Geometry check sheet. Reference: the model listing, model coordinates, mm. A direction names the side the tool comes from. Round coordinates to 2 decimals unless told otherwise and drop trailing zeros. Loops run counter-clockwise (first coordinate to the right, second up) from the corner with the lowest first, then second, coordinate; pieces in that order, holes last. Notation, with made-up numbers: M 4.25,33 L 13.25,33 A24 cw 13.25,48 Z; hole C 40,80 d7. An arc over 180 degrees is marked long. Answer in a Markdown table with one row per item. Add a question column.
```python
from build123d import *

# Parameters (mm, degrees)
F1_DEPTH = 6
F2_R     = 3
F3_DEPTH = 4.5
F5_D     = 3.5


# Not quite as in the source:
# - ends of sketch curves that miss each other by under 0.0002 mm in the source are joined


with BuildPart() as f1:
    # F0 (on Front) → F1 (new body)
    with BuildSketch(Plane.XZ):
        with BuildLine():
            Line((14.498358, 10), (14.498358, 14))
            Line((14.498358, 14), (14.498358, 14.25))
            Line((14.498358, 14.25), (15.498358, 14.25))
            Line((15.498358, 14.25), (16.539344, 12.069217))
            ThreePointArc((16.539344, 12.069217), (16.9083128035, 11.6541918591), (17.4418, 11.5))
            Line((17.4418, 11.5), (17.998358, 11.5))
            ThreePointArc((17.998358, 11.5), (18.3519113906, 11.6464466094), (18.498358, 12))
            Line((18.498358, 12), (18.498358, 24.5))
            ThreePointArc((18.498358, 24.5), (17.9125715624, 25.9142135624), (16.498358, 26.5))
            Line((16.498358, 26.5), (14.498358, 26.5))
            ThreePointArc((14.498358, 26.5), (13.0841444376, 25.9142135624), (12.498358, 24.5))
            Line((12.498358, 24.5), (12.498358, 22.5))
            Line((12.498358, 22.5), (12.498358, -16.25))
            ThreePointArc((12.498358, -16.25), (11.9125715624, -17.6642135624), (10.498358, -18.25))
            Line((10.498358, -18.25), (8.106805, -18.25))
            ThreePointArc((8.106805, -18.25), (4.9031601399, -18.5082508473), (1.7822496797, -19.276334039))
            Line((1.7822496797, -19.276334039), (-3.290569563, -20.9672737865))
            ThreePointArc((-3.290569563, -20.9672737865), (-4.8717084961, -24.1295514929), (-1.7094308537, -25.710690554))
            Line((-1.7094308537, -25.710690554), (2.709257, -24.237795))
            ThreePointArc((2.709257, -24.237795), (5.8301671399, -23.4697108473), (9.033812, -23.21146))
            Line((9.033812, -23.21146), (19.837293, -23.21146))
            ThreePointArc((19.837293, -23.21146), (20.3091070562, -22.8769637655), (20.1496410116, -22.3210259855))
            Line((20.1496410116, -22.3210259855), (16.154532, -19.124939))
            ThreePointArc((16.154532, -19.124939), (15.8900609581, -19.0948301233), (15.748358, -19.320156))
            Line((15.748358, -19.320156), (15.748358, -21.25))
            Line((15.748358, -21.25), (8.593639, -21.25))
            ThreePointArc((8.593639, -21.25), (5.3899932959, -21.5082508219), (2.2690829797, -22.276333939))
            Line((2.2690829797, -22.276333939), (-1.630813, -23.576299))
            ThreePointArc((-1.630813, -23.576299), (-2.263268599, -23.260072033), (-1.947040883, -22.627616351))
            Line((-1.947040883, -22.627616351), (2.106805, -21.276334))
            ThreePointArc((2.106805, -21.276334), (5.2277158277, -20.5082508979), (8.431361, -20.25))
            Line((8.431361, -20.25), (13.498358, -20.25))
            ThreePointArc((13.498358, -20.25), (14.2054647812, -19.9571067812), (14.498358, -19.25))
            Line((14.498358, -19.25), (14.498358, 10))
        make_face()
    extrude(amount=F1_DEPTH)

    # F2 (on face) → F3 (join)
    with BuildSketch(Plane.YZ.offset(14.498358)):
        with Locations((-3, -1.25)):
            Circle(F2_R)
    extrude(amount=F3_DEPTH)

    # F5 (through all)
    with Locations(Plane.YZ.offset(18.998358)):
        with Locations((-3, -1.25)):
            Hole(F5_D / 2)


solid = f1.part
```
1) Cross-section at B-B, the plane z = -6. Record the boundary of the cut face in (x, y).
2) Go/stop test with flat-tipped pins: pin 1 (1.8 mm diameter, centred on y = -3.5, z = 4, fed in from -X); pin 2 (3 mm diameter, centred on y = -2, z = -9, fed in from +X); pin 3 (1.5 mm diameter, centred on x = 12, y = -4, fed in from -Z); pin 4 (12 mm diameter, centred on x = 0.5, z = 0, fed in from +Y). Record where each tip stops, or that it passes through.
3) Cross-section at C-C, the plane x = 3.5. Record the boundary of the cut face in (y, z), plus the area to 3 significant figures.
4) Set-up check for faces 4 (the flat face through (14, -3, -23.211)), 5 (the flat face through (15.748, -3, -20)), 6 (the flat face through (18.18, -2.958, -20.745)): record each of +Z, -Z, +X, -X, +Y, -Y from which the full face is reachable in a straight line by a thin tool's end or side.
5) Cross-section at A-A, the plane x = 6.75. Record the boundary of the cut face in (y, z).
6) Thickness scan on L1, parallel to Z at x = 15.25, y = -3; L2, parallel to Z at x = 17.5, y = -0.4; L3, parallel to Z at x = 18.25, y = -5.05. Record the ranges inside material, lowest first. Write a range as [from, to].
7) Draft check along Z on faces 1 (the flat face through (18.998, -2, -3)), 2 (the cylindrical face through (-2.26, -2.96, -23.27)), 3 (the cylindrical face through (4.95, -2.96, -18.5)). Enter one of: +Z half, -Z half, draft (parallel to the pull), parting line (faces both ways), or undercut.
Worked answers:
| question | item | result |
|---|---|---|
| 1 | outline | M 12.5,-6 L 14.5,-6 L 14.5,0 L 12.5,0 Z |
| 2 | pin 1 | stops at x = 12.5 |
| 2 | pin 2 | stops at x = 14.5 |
| 2 | pin 3 | stops at z = -23.21 |
| 2 | pin 4 | passes through |
| 3 | outline | M -6,-23.99 L 0,-23.99 L 0,-21.91 L -6,-21.91 Z; M -6,-20.87 L 0,-20.87 L 0,-18.79 L -6,-18.79 Z |
| 3 | area | 25.0 mm2 |
| 4 | face 4 | -Z, +X, +Y, -Y |
| 4 | face 5 | +Y, -Y |
| 4 | face 6 | +X, +Y, -Y |
| 5 | outline | M -6,-23.34 L 0,-23.34 L 0,-21.34 L -6,-21.34 Z; M -6,-20.32 L 0,-20.32 L 0,-18.3 L -6,-18.3 Z |
| 6 | L1 | z = [-23.21, -21.25], [-4.25, -3], [0.5, 1.75], [14.25, 26.5] |
| 6 | L2 | z = [-23.21, -20.2], [-2.75, 0.25], [11.5, 26.23] |
| 6 | L3 | z = [-23.21, -20.8], [-3.44, 0.94], [11.57, 25.47] |
| 7 | face 1 | draft |
| 7 | face 2 | undercut |
| 7 | face 3 | +Z half |
